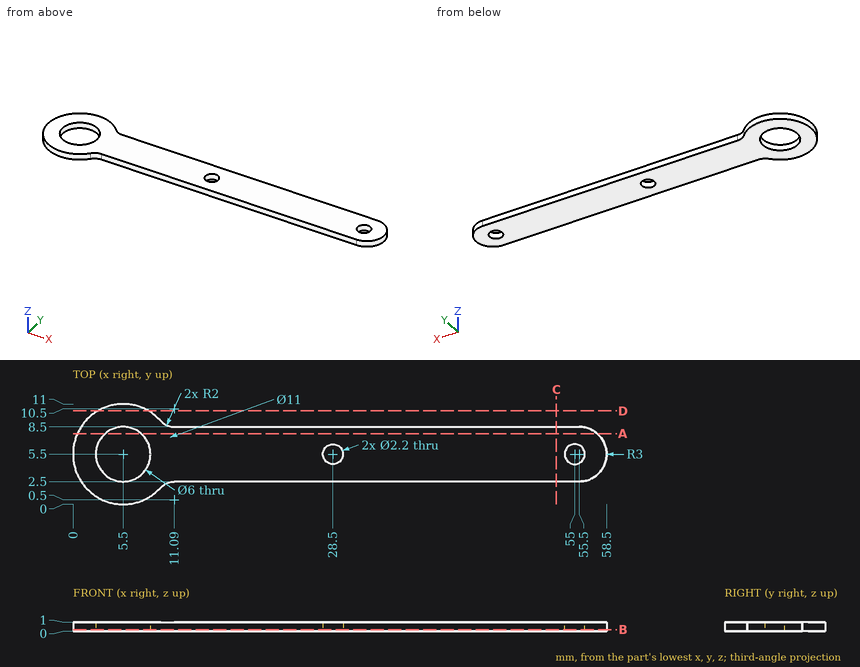
Verification items for this drawing (mm, ordinates from the low corner). Coordinates: 2 decimals unless noted, no trailing zeros. Loops run counter-clockwise (first coordinate to the right, second up) from the corner with the lowest first, then second, coordinate; pieces in that order, holes last. Notation, with made-up numbers: (82.25, 55.5) -> (138.25, 55.5) arc R15 cw to (138.25, 63.5) -> close; hole circle Ø9 at (-36, 71). An arc over 180 degrees is marked (long way). Put each result on its own line as item: value.
1. Section check A-A, the plane y = 7.75. Record the boundary of the cut face in (x, z).
Result set:
outline: (0.48, 0) -> (3.52, 0) -> (3.52, 1) -> (0.48, 1) -> close; (7.48, 0) -> (57.48, 0) -> (57.48, 1) -> (7.48, 1) -> close
2. Section check D-D, the plane y = 10.25. Record the boundary of the cut face in (x, z).
Result set:
outline: (2.73, 0) -> (8.27, 0) -> (8.27, 1) -> (2.73, 1) -> close
3. Gauge pin test, flat ends, axial feed: P1, Ø1.8, axis at x = 28.5, y = 5.5, coming from the +Z side (1 decimal); P2, Ø2.5, axis at x = 55, y = 5.5, coming from the -Z side. Record the tip position at first contact, or that the pin passes through.
Result set:
P1: passes through
P2: stops at z = 0
4. Thickness scan on line 1 (X direction, y = 5.75, z = 0.95); line 2 (Y direction, x = 55, z = 0.25); line 3 (Y direction, x = 51, z = 0.8). Record the ranges inside material, lowest first.
Result set:
line 1: x = 0.01 to 2.51, 8.49 to 27.43, 29.57 to 53.93, 56.07 to 58.49
line 2: y = 2.5 to 4.4, 6.6 to 8.5
line 3: y = 2.5 to 8.5
5. Section check C-C, the plane x = 53. Record the boundary of the cut face in (y, z).
Result set:
outline: (2.5, 0) -> (8.5, 0) -> (8.5, 1) -> (2.5, 1) -> close
6. Section check B-B, the plane z = 0.2. Record the boundary of the cut face in (x, y), then the cut area to 3 significant figures.
Result set:
outline: (9.6, 1.83) arc R2 cw to (11.09, 2.5) -> (55.5, 2.5) arc R3 ccw to (55.5, 8.5) -> (11.09, 8.5) arc R2 cw to (9.6, 9.17) arc R5.5 ccw (long way) to start; hole circle Ø6 at (5.5, 5.5); hole circle Ø2.2 at (28.5, 5.5); hole circle Ø2.2 at (55, 5.5)
area: 342 mm^2
